Build history of the part. All positions in model axes, mm. Round coordinates to 2 decimals unless told otherwise and drop trailing zeros. Order: outer loops, then holes, each group sorted by start corner. A loop starts at its lowest first (then second) coordinate and runs counter-clockwise, first axis right, second up. Notation, with made-up numbers: (66, 38.25) -> (109, 38.25) arc R12 ccw to (109, 58.25) -> close; hole circle Ø5 at (-3, -15). An arc over 180 degrees is marked (long way). Write item = value, one per line.
from build123d import *

# Parameters (mm, degrees)
F0_W     = 150
F0_H     = 150
F0_R     = 3
F0_R_2   = 11.5
F1_DEPTH = 7
F2_SIZE  = 5
F3_R     = 5


with BuildPart() as f1:
    # F0 (on Front) → F1 (new body)
    with BuildSketch(Plane.XZ):
        Rectangle(F0_W, F0_H)
        with Locations((-55, -55)):
            Circle(F0_R, mode=Mode.SUBTRACT)
        with Locations((55, -55)):
            Circle(F0_R, mode=Mode.SUBTRACT)
        with Locations((-55, 55)):
            Circle(F0_R, mode=Mode.SUBTRACT)
        Circle(F0_R_2, mode=Mode.SUBTRACT)
        with Locations((55, 55)):
            Circle(F0_R, mode=Mode.SUBTRACT)
    extrude(amount=F1_DEPTH)

    # F2
    f2_edges = [f1.edges().sort_by_distance(p)[0] for p in [
        (-11.5, 0, 0),
    ]]
    chamfer(f2_edges, length=F2_SIZE)

    # F3
    f3_edges = [f1.edges().sort_by_distance(p)[0] for p in [
        (75, -3.5, 75),
        (-75, -3.5, 75),
        (-75, -3.5, -75),
        (75, -3.5, -75),
    ]]
    fillet(f3_edges, radius=F3_R)


solid = f1.part
Q1. Cut at C-C, the plane z = -55. List the corners of the cut face in (x, y).
Check values:
outline = (-75, -7) -> (-58, -7) -> (-58, 0) -> (-75, 0) -> close; (-52, -7) -> (52, -7) -> (52, 0) -> (-52, 0) -> close; (58, -7) -> (75, -7) -> (75, 0) -> (58, 0) -> close
Q2. Cut at D-D, the plane x = 55. List the corners of the cut face in (y, z).
Check values:
outline = (-7, -75) -> (0, -75) -> (0, -58) -> (-7, -58) -> close; (-7, -52) -> (0, -52) -> (0, 52) -> (-7, 52) -> close; (-7, 58) -> (0, 58) -> (0, 75) -> (-7, 75) -> close
Q3. Probe probe 1 along Z at (x, y) = (55, -6.25); probe 2 along Z at (x, y) = (57, -0.75). List the from-to ranges inside material, lowest first.
Check values:
probe_1 = -75 to -58, -52 to 52, 58 to 75
probe_2 = -75 to -57.24, -52.76 to 52.76, 57.24 to 75
Q4. Flat gauge pin, fed straight in: pin 1 (5.5 mm diameter, centred on x = 55, z = 55, fed in from +Y). Where does the tip first touch, or does it go through?
Check values:
pin_1 = through
Q5. Mould opens along X. For faces 1 (the face through (-74, -4, 73)), 2 (the face through (73, -4, -74)), 3 (the face through (-1, -3, -75)), 4 (the face through (-57.21, -3.45, -52.97)) say: released by +X, released by -X, zero draft, split by the parting line, or undercut.
Check values:
face_1 = released by -X
face_2 = released by +X
face_3 = zero draft
face_4 = undercut
Q6. Cut at B-B, the plane z = 0. List the corners of the cut face in (x, y).
Check values:
outline = (-75, -7) -> (-11.5, -7) -> (-11.5, -5) -> (-16.5, 0) -> (-75, 0) -> close; (11.5, -7) -> (75, -7) -> (75, 0) -> (16.5, 0) -> (11.5, -5) -> close
Q7. Cut at A-A, the plane x = 0. List the corners of the cut face in (y, z), and give its area (3 significant figures).
Check values:
outline = (-7, -75) -> (0, -75) -> (0, -16.5) -> (-5, -11.5) -> (-7, -11.5) -> close; (-7, 11.5) -> (-5, 11.5) -> (0, 16.5) -> (0, 75) -> (-7, 75) -> close
area = 864 mm²
